Here's the drawing with two shaded views (mm, measured from the low corner). I have some questions. A direction names the side the tool comes from. Give positions to 0.01 mm unless a question says otherwise; leave off trailing zeros. Write each loop counter-clockwise with the first axis right and the second up, starting at its lowest first coordinate (ties: lowest second). Pieces come first, ordered by that corner, then holes. Notation, with made-up numbers: (66.5, 39.5) - (115.5, 39.5) arc R3 cw to (115.5, 44.5) - close; hole circle Ø4 at (9, -7.75). An arc over 180 degrees is marked (long way). Use one line per item in the form item = value.
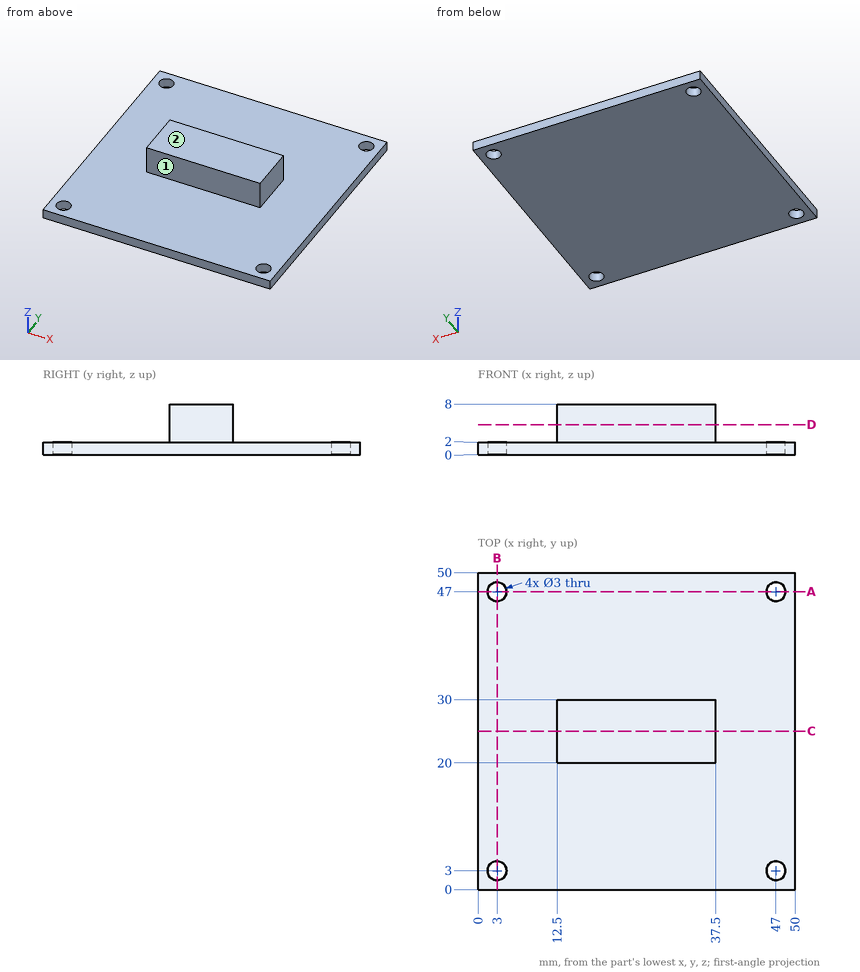
1. Imagine slicing it at C-C, the plane y = 25. List the corners of the cut face in (x, z) for me.
Response values:
outline = (0, 0) - (50, 0) - (50, 2) - (37.5, 2) - (37.5, 8) - (12.5, 8) - (12.5, 2) - (0, 2) - close
2. Imagine slicing it at D-D, the plane z = 4.75. List the corners of the cut face in (x, y) for me, and give its area (3 significant figures).
Response values:
outline = (12.5, 20) - (37.5, 20) - (37.5, 30) - (12.5, 30) - close
area = 250 mm²
3. For pin 1 (1.8 mm diameter, centred on y = 22.5, z = 5.5, fed in from +X); pin 2 (3.5 mm diameter, centred on x = 47, y = 3, fed in from +Z); pin 3 (4 mm diameter, centred on x = 30.5, z = 6, fed in from +Y), each with a flat end and sliding along its axis, tell me the tip position at first contact or that it passes through.
Response values:
pin_1 = 37.5
pin_2 = 2
pin_3 = 30
4. Imagine slicing it at A-A, the plane y = 47. List the corners of the cut face in (x, z) for me.
Response values:
outline = (0, 0) - (1.5, 0) - (1.5, 2) - (0, 2) - close; (4.5, 0) - (45.5, 0) - (45.5, 2) - (4.5, 2) - close; (48.5, 0) - (50, 0) - (50, 2) - (48.5, 2) - close
5. If I drill on line 1 (X direction, y = 47, z = 1.15); line 2 (Y direction, x = 31, z = 5.5), over which ranges is the centre line in solid material (lowest first)? Write a range as from..to.
Response values:
line_1 = 0..1.5, 4.5..45.5, 48.5..50
line_2 = 20..30
6. Which directions (+Z, -Z, +X, -X, +Y, -Y) give clear straight access to the entire face, cutting with the end or side of a thin tool? Please do the marked faces 1 and 2.
Response values:
face_1 = +Z, +X, -X, -Y
face_2 = +Z, +X, -X, +Y, -Y
